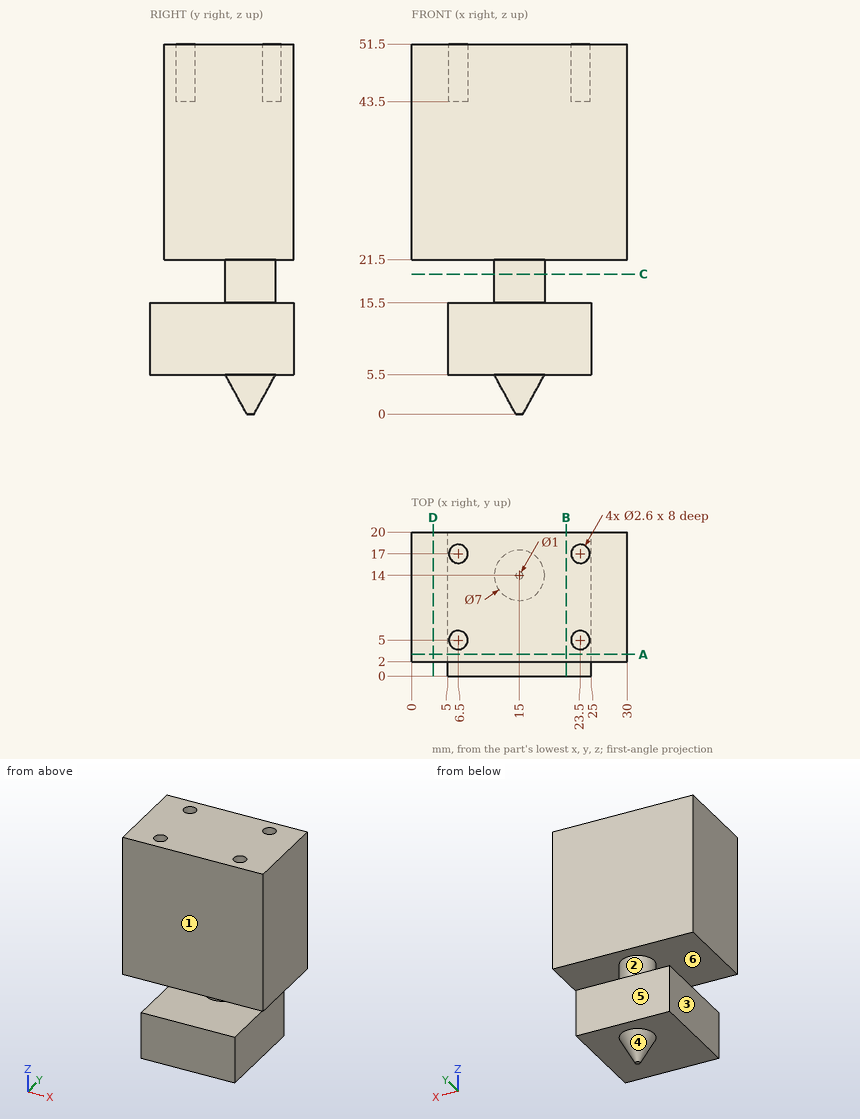
Geometry: see drawing. Coordinates: mm, zero at the bounding-box minimum. A direction names the side the tool comes from. Round coordinates to 2 decimals unless told otherwise and drop trailing zeros. Loops run counter-clockwise (first coordinate to the right, second up) from the corner with the lowest first, then second, coordinate; pieces in that order, holes last. Notation, with made-up numbers: (48, 83) -> (95, 83) arc R24 cw to (95, 96) -> close; hole circle Ø4 at (-30.75, -7). An arc over 180 degrees is marked (long way). Use one line per item in the form item = value. Start each with the question number.
Item 1: Section query C-C on z = 19.5. Return the cut outline in (x, y), then the cut area to 3 significant figures.
Item 2: Contact query for flat-ended pins moving along their axis: pin 1 Ø12 at (x, y) = (18, 8) entering from -Z; pin 2 Ø1.5 at (x, y) = (6, 14.5) entering from -Z; pin 3 Ø15 at (x, z) = (13.5, 30.5) entering from -Y. Output: stop coordinate, or through.
Item 3: Material intervals for L1, parallel to Y at x = 6.5, z = 48.5; L2, parallel to Z at x = 17.5, y = 9; L3, parallel to Y at x = 2, z = 26.5, sorted ascending. Write a range as from..to.
Item 4: Section query D-D on x = 3. Return the cut outline in (y, z), then the cut area to 3 significant figures.
Item 5: Section query B-B on x = 21.5. Return the cut outline in (y, z), then the cut area to 3 significant figures.
Item 6: Section query A-A on y = 3. Return the cut outline in (x, z).
Item 7: Mould query, pull axis Z, two halves, no side actions, for the marked faces 4, 5 and 6. Classes: pulls with the +Z half, pulls with the -Z half, needs draft (parallel to the pull), parting line crosses it, or undercut.
Item 8: Set-up query: the marked faces 1, 2 and 3. Return all of +Z, -Z, +X, -X, +Y, -Y with unobstructed straight access to the full face (end or side cutting, diameter ignored); none if empty.
Ans:
q1.outline = circle Ø7 at (15, 14)
q1.area = 38.5 mm^2
q2.pin_1 = 0.38
q2.pin_2 = 5.5
q2.pin_3 = 2
q3.L1 = 2..3.7, 6.3..15.7, 18.3..20
q3.L2 = 5.5..15.5, 21.5..51.5
q3.L3 = 2..20
q4.outline = (2, 21.5) -> (20, 21.5) -> (20, 51.5) -> (2, 51.5) -> close
q4.area = 540 mm^2
q5.outline = (0, 5.5) -> (20, 5.5) -> (20, 15.5) -> (0, 15.5) -> close; (2, 21.5) -> (20, 21.5) -> (20, 51.5) -> (2, 51.5) -> close
q5.area = 740 mm^2
q6.outline = (0, 21.5) -> (30, 21.5) -> (30, 51.5) -> (0, 51.5) -> close; (5, 5.5) -> (25, 5.5) -> (25, 15.5) -> (5, 15.5) -> close
q7.face_4 = pulls with the -Z half
q7.face_5 = needs draft
q7.face_6 = undercut
q8.face_1 = +Z, +X, -X, -Y
q8.face_2 = none
q8.face_3 = -Z, -X, +Y, -Y
